Can you work these out from the drawing? Everything is in mm from the part's minimum corner. A direction names the side the tool comes from. Round coordinates to 2 decimals unless told otherwise and drop trailing zeros. Order: outer loops, then holes, each group sorted by start corner. A loop starts at its lowest first (then second) coordinate and runs counter-clockwise, first axis right, second up. Notation, with made-up numbers: (31, 55) -> (69, 55) arc R6 cw to (69, 66) -> close; hole circle Ø11 at (46.5, 50). An arc over 180 degrees is marked (long way). One line per item, written item: value.
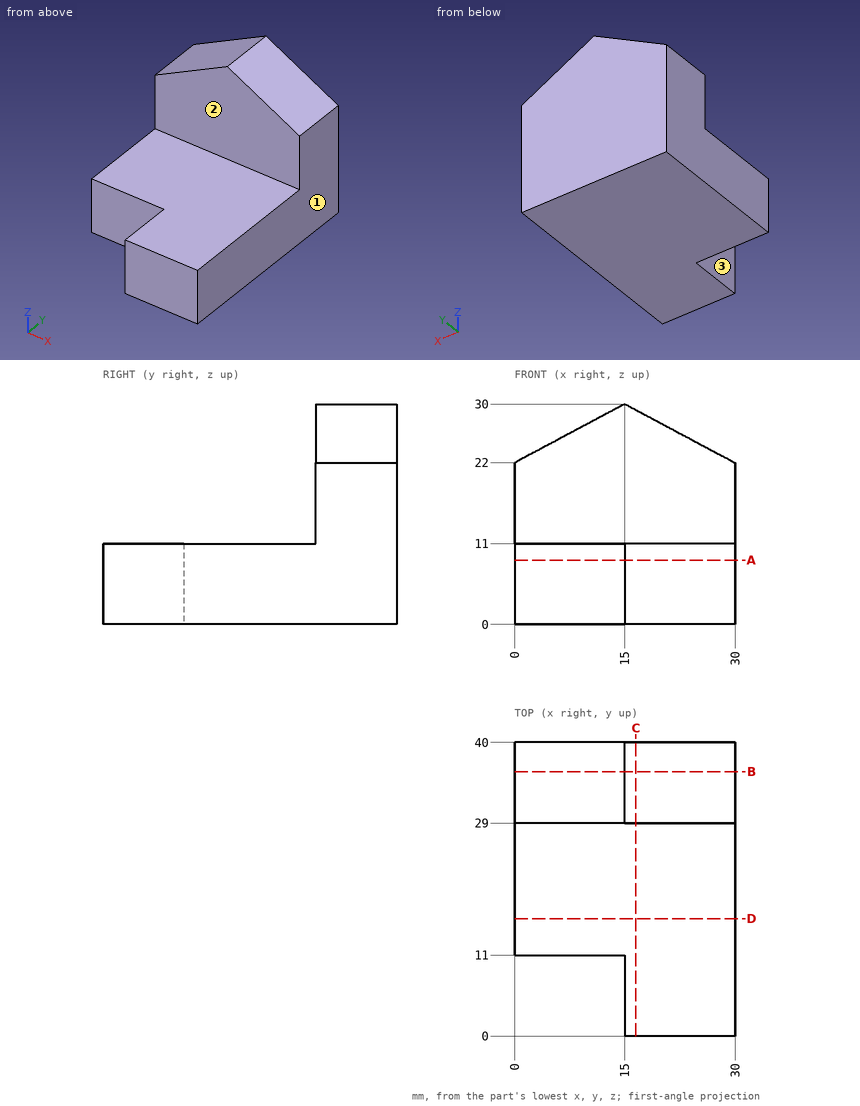
Q1. I want a section at D-D on y = 16. Write out the boundary of the cut face in (x, z), then the cut area to 3 significant figures.
Answers:
outline: (0, 0) -> (30, 0) -> (30, 11) -> (0, 11) -> close
area: 330 mm2
Q2. I want a section at A-A on z = 8.75. Write out the boundary of the cut face in (x, y), then the cut area to 4 significant figures.
Answers:
outline: (0, 11) -> (15, 11) -> (15, 0) -> (30, 0) -> (30, 40) -> (0, 40) -> close
area: 1,035 mm2
Q3. I want a section at C-C on x = 16.5. Write out the boundary of the cut face in (y, z), then the cut area to 3 significant figures.
Answers:
outline: (0, 0) -> (40, 0) -> (40, 29.2) -> (29, 29.2) -> (29, 11) -> (0, 11) -> close
area: 640 mm2
Q4. I want a section at B-B on y = 36. Write out the boundary of the cut face in (x, z).
Answers:
outline: (0, 0) -> (30, 0) -> (30, 22) -> (15, 30) -> (0, 22) -> close
Q5. For P1, Ø1, axis at y = 9, z = 13, coming from the -X side; P2, Ø5, axis at x = 6.5, z = 21, coming from the -Y side; P3, Ø5, axis at x = 12, y = 14.5, coming from the +Z side; P4, Ø9, axis at x = 7.5, z = 7.5, coming from the -Y side, each with a flat end and sliding along its axis, tell me the tip position at first contact or that it passes through.
Answers:
P1: through
P2: y = 29
P3: z = 11
P4: y = 11
Q6. I need wall thicknesses on line 1 along Y through (x, z) = (12, 23); line 2 along Y through (x, z) = (9.5, 10.5); line 3 along Z through (x, y) = (27, 26). Which ranges of each line are inside material? Lowest first, please.
Answers:
line 1: 29 to 40
line 2: 11 to 40
line 3: 0 to 11
Q7. Which directions (+Z, -Z, +X, -X, +Y, -Y) give clear straight access to the entire face, cutting with the end or side of a thin tool? Please do the marked faces 1, 2 and 3.
Answers:
face 1: +Z, -Z, +X, +Y, -Y
face 2: +Z, +X, -X, -Y
face 3: +Z, -Z, -X, -Y
